Can you work these out from the model? Positions are in its coordinate system, mm. A direction names the side the tool comes from. Round coordinates to 2 decimals unless told otherwise and drop trailing zeros. Loops run counter-clockwise (first coordinate to the right, second up) from the corner with the lowest first, then second, coordinate; pieces in that order, holes last. Notation, with made-up numbers: M 44,-27.75 L 59,-27.75 A24 ccw 59,-3.75 Z; hole C 7.25,-37.75 d1. An arc over 180 degrees is marked long. Answer as CSV lines item,"result".
Autodesk Inventor part; units mm, degrees
ref_plane "YZ Plane" through (0, 0, 0) normal (1, 0, 0) x (0, 1, 0)
ref_plane "XZ Plane" through (0, 0, 0) normal (0, 1, 0) x (-1, 0, 0)
ref_plane "XY Plane" through (0, 0, 0) normal (0, 0, 1) x (1, 0, 0)
sketch "Sketch1" plane through (0, 0, 0) normal (0, 0, 1) x (1, 0, 0)
  line L0 (16.0355, 8.5355) -> (20.0355, 8.5355)
  line L1 (-73.9645, 8.5355) -> (16.0355, 8.5355)
  line L2 (20.0355, 8.5355) -> (-73.9645, 8.5355)
  line L3 (-73.9645, 27.5374) -> (-73.9645, 23.5355)
  line L4 (40.7522, 23.5355) -> (40.7524, 27.5)
  line L5 (20.0355, 8.5355) -> (20.0355, 12.5391)
  line L6 (40.7522, 12.5355) -> (40.7527, 27.5355)
  line L7 (-73.9639, 27.5391) -> (-73.9643, 12.5391)
  line L8 (-73.9636, 27.541) -> (40.7527, 27.5355)
  line L9 (-73.9643, 12.5391) -> (-73.9636, 27.541)
  line L10 (-77.7958, 27.5374) -> (-77.7958, 31.5374)
  line L11 (-77.7958, 31.5374) -> (-73.7958, 31.5374)
  line L12 (-73.7958, 31.5374) -> (40.9206, 31.5374)
  line L13 (40.9206, 31.5374) -> (44.7523, 31.5374)
  line L14 (44.7523, 27.5355) -> (44.7523, 31.5374)
  line L15 (-77.7958, 27.5374) -> (-77.7958, 8.5355)
  line L16 (-77.7958, 3.9889) -> (-77.7958, 8.5355)
  line L17 (44.7115, 3.9884) -> (44.7523, 8.5718)
  line L18 (-14.4375, 3.9889) -> (-21.9375, 3.9889)
  line L19 (-21.9375, 3.9889) -> (-6.9375, 3.9889)
  line L20 (-6.9375, 3.9889) -> (-6.9375, -15.0111)
  line L21 (-6.9375, -15.0111) -> (-21.9375, -15.0111)
  line L22 (-21.9375, -15.0111) -> (-21.9375, 3.9889)
  line L23 (-23.9375, -15.0111) -> (-23.9375, -17.0111)
  line L24 (-4.9375, -17.0111) -> (-4.9375, 5.9889)
  line L25 (-4.9375, 5.9889) -> (-23.9375, 5.9889)
  line L26 (-23.9375, 5.9889) -> (-23.9375, -17.0111)
  line L27 (-23.9375, -21.0111) -> (-77.7958, -21.0111)
  line L28 (-77.7958, -21.0111) -> (-77.7958, 3.9889)
  line L29 (-73.9645, 8.5355) -> (-73.9645, -17.0111)
  line L30 (-73.9645, -17.0111) -> (-23.9375, -17.0111)
  line L31 (-23.9375, -21.0111) -> (-4.9375, -21.0111)
  line L32 (-4.9375, -21.0111) -> (44.7115, -21.0111)
  line L33 (44.7115, -21.0111) -> (44.7115, 3.9884)
  line L34 (40.7522, 8.5355) -> (40.7522, -17.0111)
  line L35 (40.7522, -17.0111) -> (-4.9375, -17.0111)
  line L36 (-73.9643, 12.5391) -> (20.0355, 12.5391)
  line L37 (-73.9645, 8.5355) -> (20.0355, 8.5355)
  line L38 (40.7522, 12.5355) -> (40.7522, 8.5355)
  line L39 (44.7523, 27.5355) -> (44.7523, 8.5718)
  line L40 (-23.9375, -17.0111) -> (-4.9375, -17.0111)
  point P0 (0, 0)
  point P1 (-73.9645, 27.5355)
  point P2 (40.7521, 27.5)
extrude "Extrusion1" add sketch "Sketch1" against normal blind 4 contours L0 L5 L36 L7 L3 L9 L8 L6 L4 L38 L34 L35 L24 L25 L26 L23 L30 L29 L1 | L23 L26 L25 L24 L40 | L10 L11 L12 L13 L14 L39 L17 L33 L32 L31 L27 L28 L16 L15 | L19 L20 L21 L22 L18
extrude "Extrusion2" add sketch "Sketch1" along normal blind 75 contours L10 L11 L12 L13 L14 L39 L17 L33 L32 L31 L27 L28 L16 L15
sketch "Sketch3" plane through (0, 0, 0) normal (0, 0, 1) x (1, 0, 0)
  line L0 (-73.9645, -21.4645) -> (40.7521, -21.4645)
  line L1 (40.7521, -21.4645) -> (29.7521, -21.4645)
  line L2 (29.7521, -21.4645) -> (29.7521, -3.4645)
  line L3 (29.7521, -3.4645) -> (40.7521, -3.4645)
  line L4 (40.7521, -3.4645) -> (40.7521, -21.4645)
  circle A0 centre (29.7521, -3.4645) radius 2.5
  point P0 (0, 0)
  dimension "d44" = 11
  dimension "d45" = 18
  dimension "d46" = 5
extrude "Extrusion5" cut sketch "Sketch3" against normal blind 4 contours A0 L3 L2 | L2 L3 A0
extrude "Extrusion8" add sketch "Sketch1" along normal blind 35 contours L23 L26 L25 L24 L40
extrude "Extrusion9" add sketch "Sketch1" along normal blind 34 contours L19 L20 L21 L22 L18
sketch "Sketch6" plane through (-73.9645, -17.0111, 75) normal (0, 1, 0) x (1, 0, 0)
  line L0 (69.0269, 40) -> (50.0269, 40)
  line L1 (50.0269, 40) -> (69.0269, 40)
  line L2 (69.0269, 75) -> (69.0269, 40)
  circle A0 centre (59.5269, 35.25) radius 4.75
  circle A1 centre (59.5269, 35.25) radius 5.75
  point P0 (73.9645, 75)
  dimension "d71" = 11.5
extrude "Extrusion10" cut sketch "Sketch6" against normal blind 4 contours A0
extrude "Extrusion11" add sketch "Sketch6" against normal blind 14
sketch "Sketch7" plane through (44.7115, 3.9884, 75) normal (1, -0.0089, 0) x (0, 0, -1)
  line L0 (79, -26.0867) -> (0, -26.0867)
  line L1 (79, 26.4598) -> (79, 27.5484)
  line L2 (0, -26.0867) -> (79, -26.0867)
  line L3 (79, -26.0867) -> (79, 27.5484)
  line L4 (79, 27.5484) -> (0, 27.5484)
  line L5 (0, 27.5484) -> (0, -26.0867)
  line L6 (0, 0.7308) -> (79, 0.7308)
  line L7 (39.5, -26.0867) -> (39.5, 27.5484)
  circle A0 centre (39.5, 0.7308) radius 2.3
  circle A1 centre (39.5, 0.7308) radius 3.3
  line L8 (39.5, -2.5692) -> (79, -2.5692)
  line L9 (39.5, 4.0308) -> (79, 4.0308)
  point P0 (75, -4.3854)
  dimension "d76" = 4.6
  dimension "d77" = 6.6
extrude "Extrusion12" add sketch "Sketch7" along normal blind 6 contours L8 A1 L6 L3 | A1 L6 A0 L7 | L7 A0 L6 A1 | L6 A1 L9 L3 | L6 A0 L7 A1 | A1 L7 A0 L6
sketch "Sketch8" plane through (-77.7958, -21.0111, -4) normal (-1, 0, 0) x (0, 0, 1)
  line L0 (0, 0) -> (79, 0)
  line L1 (79, 52.5485) -> (0, 52.5485)
  line L2 (0, 52.5485) -> (0, 0)
  line L3 (0, 0) -> (79, 0)
  line L4 (79, 0) -> (79, 52.5485)
  line L5 (0, 52.5485) -> (79, 52.5485)
  line L6 (39.5, 52.5485) -> (39.5, 0)
  line L7 (42.7181, 24.9994) -> (79, 24.9994)
  line L8 (79, 24.9994) -> (0, 25.6769)
  line L9 (0, 22.3771) -> (0, 28.9768)
  circle A0 centre (39.5, 25.6768) radius 2.3
  ellipse E0 centre (39.5, 25.6769) end of major axis (41.8, 25.6769) minor radius 2.2999
  circle A1 centre (39.5, 25.6768) radius 3.3
  line L10 (39.5, 28.9768) -> (0, 28.9768)
  line L11 (39.5, 22.3768) -> (0, 22.3771)
  point P0 (4, 21.0111)
  dimension "d80" = 6.6
extrude "Extrusion13" add sketch "Sketch8" along normal blind 6 contours L2 L8 A1 L11 | A1 L8 A0 L6 | L6 A0 L8 A1 | L2 L10 A1 L8 | A1 L6 A0 L8 | L8 A0 L6 A1
properties part number "Bakje sensor" material "ABS Plastic"
Item 1: On a 3-axis mill with a long thin cutter (end or side, diameter ignored), from which of +Z, -Z, +X, -X, +Y, -Y can I reach the whole of each face in a straight line? I mean faces 1 (the face through (-80.8, 4.7, 38.8)), 2 (the face through (-15.06, -23.91, 35.04)), 3 (the face through (-83.796, 5, 17)), 4 (the face through (-4.938, -6, 17)). Say none if no direction works.
Output:
face 1,"+Z, -X"
face 2,"-Y"
face 3,"+Z, -Z, -X, +Y, -Y"
face 4,"+Z"
Item 2: If I drill on line 1 along Y through (x, z) = (-54, 58); line 2 along X through (y, z) = (-5.5, 4); line 3 along X through (y, z) = (5, 15.5), over which ranges is the centre line in solid material (lowest first)? Write a range as from..to.
Output:
line 1,"y = -21.01..-17.01, 8.54..12.54, 27.54..31.54"
line 2,"x = -77.8..-73.96, -23.94..-4.94, 40.75..44.71"
line 3,"x = -83.8..-73.96, -23.94..-4.94, 40.75..50.72"
Item 3: If we section it at C-C on x = -58: Write out the boundary of the cut face in (y, z), then the cut area to 3 significant figures.
Output:
outline,"M -21.01,-4 L 31.54,-4 L 31.54,75 L 27.54,75 L 27.54,0 L 12.54,0 L 12.54,75 L 8.54,75 L 8.54,0 L -17.01,0 L -17.01,75 L -21.01,75 Z"
area,"1,110 mm2"
Item 4: If we section it at B-B on y = -11.5: Write out the boundary of the cut face in (x, z).
Output:
outline,"M -77.8,-4 L 44.71,-4 L 44.71,75 L 40.75,75 L 40.75,0 L -4.94,0 L -4.94,35 L -6.94,35 L -6.94,34 L -21.94,34 L -21.94,35 L -23.94,35 L -23.94,0 L -73.96,0 L -73.96,75 L -77.8,75 Z"
Item 5: We'd pull the mould along Z, two halves only. Please class faces 5 (the face through (44.752, 20, 35)), 6 (the face through (-77.796, 5, 35)), 7 (the face through (-23, -5, 35)), 8 (the face through (47.67, 4.002, 33.306)): released by +Z, released by -Z, zero draft, split by the parting line, or undercut.
Output:
face 5,"zero draft"
face 6,"undercut"
face 7,"released by +Z"
face 8,"undercut"
Item 6: Will these pins go through, and if not, where does the flat tip stop? pin 1 (2 mm diameter, centred on x = 28.5, z = 4, fed in from -Y); pin 2 (3 mm diameter, centred on y = 25, z = 30, fed in from -X); pin 3 (4 mm diameter, centred on x = 29.75, y = -3.46, fed in from +Z); pin 4 (18.5 mm diameter, centred on y = -5.5, z = 13, fed in from +X).
Output:
pin 1,"stops at y = -21.01"
pin 2,"stops at x = -77.8"
pin 3,"passes through"
pin 4,"stops at x = 50.71"
